Here's how the part is built. I have some questions about the finished solid (model axes, mm). A direction names the side the tool comes from. Coordinates: 2 decimals unless noted, no trailing zeros. Write each loop counter-clockwise with the first axis right and the second up, starting at its lowest first coordinate (ties: lowest second). Pieces come first, ordered by that corner, then holes.
Item 1: I want a section at B-B (x = 97.5). Please give me the cut outline in (y, z) (3 decimals), and give its area (3 significant figures).
Item 2: I want a section at A-A (y = -53). Please give me the cut outline in (x, z) (3 decimals), and give its area (3 significant figures).
Item 3: Please list where these lines run through material, in increasing order: line 1 (Y direction, x = 30.5, z = 45.5); line 2 (X direction, y = 23, z = 12) (3 decimals); line 3 (X direction, y = 55, z = 6) (3 decimals).
Item 4: I'm going to push flat-ended pins straight in: P1, Ø8.5, axis at y = -17.5, z = 21, coming from the -X side (3 decimals); P2, Ø2, axis at x = 22.5, z = 30, coming from the -Y side; P3, Ø18.5, axis at y = -12.5, z = 9, coming from the +X side (3 decimals). Where does each tip first touch, or does it pass through?
Item 5: If we mould it in two halves opening along X, with no side actions, what happens to faces 6 (the face through (39.365, -61.689, 0.133)), 7 (the face through (45.8, -0.4, 38.1)), 8 (the face through (30.65, 16.55, 49.75)), 9 (the face through (60, 2, 61.925))? For each: pulls with the +X half, pulls with the -X half, needs draft (parallel to the pull), parting line crosses it, or undercut.
Item 6: For faces 1 (the face through (-39.464, -61.59, -0.133)), 2 (the face through (-1, -1, -9.525)), 3 (the face through (46, -25.4, 42)), 4 (the face through (41.275, -1, 4)), 5 (the face through (-5, 7.938, 30)), which set-ups out of +Z, -Z, +X, -X, +Y, -Y let a thin tool reach every point of the face, with its end or its side?
from build123d import *

# Parameters (mm, degrees)
F1_DEPTH = 63.5
F2_DEPTH = 25.4
F0_W     = 25.4
F0_H     = 19.05
F3_DEPTH = 25.4
F5_DEPTH = 7.9375
F6_R     = 6.35


with BuildPart() as f1:
    # F0 (on Front) → F1 (new body, symmetric)
    with BuildSketch(Plane.XZ):
        Polygon((22.225, 9.525), (-41.275, 9.525), (-41.275, -9.525), (41.275, -9.525), (41.275, 9.525), align=None)
    extrude(amount=F1_DEPTH, both=True)

    # F0 (on Front) → F2 (join, symmetric)
    with BuildSketch(Plane.XZ):
        with BuildLine():
            Line((22.225, 27.0002), (22.225, 9.525))
            Line((22.225, 9.525), (41.275, 9.525))
            Line((41.275, 9.525), (41.275, 27.0002))
            ThreePointArc((41.275, 27.0002), (45.9246798487, 38.2255201513), (57.15, 42.8752))
            Line((57.15, 42.8752), (60.325, 42.8752))
            Line((60.325, 42.8752), (60.325, 61.9252))
            Line((60.325, 61.9252), (57.15, 61.9252))
            add(Edge.make_bspline(
                [(51.1919194088, 61.4132338777), (53.1588989286, 61.6071240271), (55.1452560975, 61.7777078906), (57.15, 61.9252)],
                knots=[106.8067988555, 106.8067988555, 106.8067988555, 106.8067988555, 111.5045361635, 111.5045361635, 111.5045361635, 111.5045361635], degree=3))
            ThreePointArc((51.1919194088, 61.4132338777), (30.4307036989, 49.4909721116), (22.225, 27.0002))
        make_face()
    extrude(amount=F2_DEPTH, both=True)

    # F0 (on Front) → F3 (join, symmetric)
    with BuildSketch(Plane.XZ):
        with Locations((73.025, 52.4002)):
            Rectangle(F0_W, F0_H)
    extrude(amount=F3_DEPTH, both=True)

    # F0 (on Front) → F4 (revolve)
    with BuildSketch(Plane.XZ):
        Polygon((85.725, 66.675), (85.725, 61.9252), (85.725, 42.8752), (85.725, 38.1), (111.125, 38.1), (111.125, 66.675), align=None)
    revolve(axis=Axis((85.725, 0, 52.3875), (0, 0, 1)))

    # F0 (on Front) → F5 (join, symmetric)
    with BuildSketch(Plane.XZ):
        with BuildLine():
            add(Edge.make_bspline(
                [(-41.275, 9.525), (-28.2331469097, 40.5493377049), (6.4710735747, 57.0049869219), (51.1919194088, 61.4132338777)],
                knots=[0, 0, 0, 0, 106.8067988555, 106.8067988555, 106.8067988555, 106.8067988555], degree=3))
            Line((-41.275, 9.525), (22.225, 9.525))
            Line((22.225, 9.525), (22.225, 27.0002))
            ThreePointArc((22.225, 27.0002), (30.4307036989, 49.4909721116), (51.1919194088, 61.4132338777))
        make_face()
    extrude(amount=F5_DEPTH, both=True)

    # F6
    f6_edges = [f1.edges().sort_by_distance(p)[0] for p in [
        (-41.275, -63.5, 0),
        (41.275, -63.5, 0),
        (41.275, 63.5, 0),
        (-41.275, 63.5, 0),
    ]]
    fillet(f6_edges, radius=F6_R)


solid = f1.part
Answer:
1. outline: (-22.506, 38.1) - (22.506, 38.1) - (22.506, 66.675) - (-22.506, 66.675) - close
1. area: 1,290 mm2
2. outline: (-41.275, -9.525) - (41.275, -9.525) - (41.275, 9.525) - (-41.275, 9.525) - close
2. area: 1,570 mm2
3. line 1: y = -25.4 to 25.4
3. line 2: x = 22.225 to 41.275
3. line 3: x = -41.275 to 41.275
4. P1: stops at x = 22.225
4. P2: stops at y = -25.4
4. P3: stops at x = 41.275
5. face 6: pulls with the +X half
5. face 7: undercut
5. face 8: pulls with the -X half
5. face 9: needs draft
6. face 1: +Z, -Z, -X, -Y
6. face 2: -Z, +X, -X, +Y, -Y
6. face 3: +Z, +X, -X, -Y
6. face 4: -Z, +X, +Y, -Y
6. face 5: +Z, -X, +Y
